The drawing under review shows one solid part. Ordinate dimensions are in mm from its lowest x, y, z. Coordinates: 2 decimals unless noted, no trailing zeros. Write each loop counter-clockwise with the first axis right and the second up, starting at its lowest first coordinate (ties: lowest second). Pieces come first, ordered by that corner, then holes.
Q1. Take a section at A-A (z = 10). Give the boundary of the cut face in (x, y), and give its area (3 significant figures).
Q2. Insertion check: pin 1 (3.5 mm diameter, centred on x = 10, z = 17, fed in from +Y); pin 2 (2.5 mm diameter, centred on x = 3, z = 10, fed in from +Y) (3 decimals). Each pin has a flat end and moves straight along its axis. Give the tip position at first contact, or say it passes through.
Q3. Mouldability with a two-part tool opening along Z and no side actions: class the marked faces 1, 2 and 3 as pulls with the +Z half, pulls with the -Z half, needs draft (parallel to the pull), parting line crosses it, or undercut.
Q4. Take a section at C-C (x = 10). Give the boundary of the cut face in (y, z).
Q5. Take a section at B-B (x = 17). Give the boundary of the cut face in (y, z), and give its area (3 significant figures).
Q6. Take a section at D-D (y = 1.5). Give the boundary of the cut face in (x, z).
Q7. For probe 1 along X at (y, z) = (1.5, 10); probe 2 along X at (y, z) = (1.45, 17.25), list the stretches that pass through material, from the lowest coordinate up.
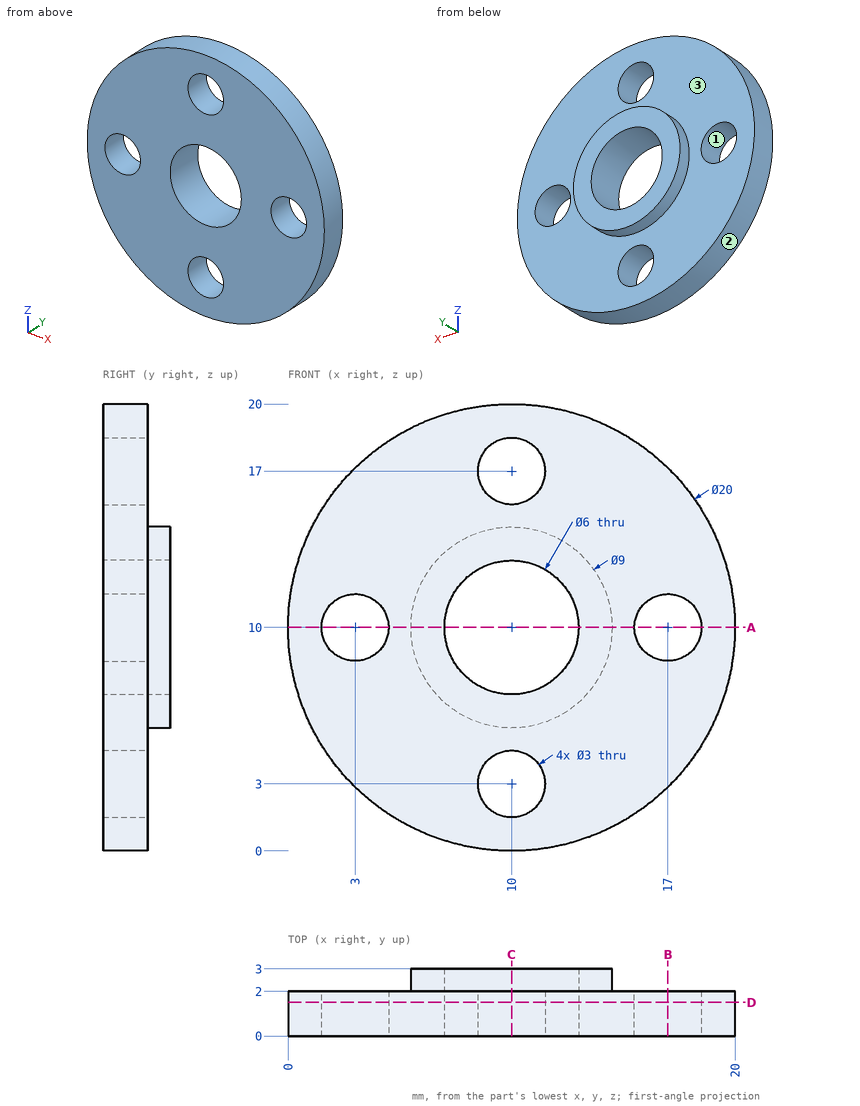
Response:
1. outline: (0, 0) - (1.5, 0) - (1.5, 2) - (0, 2) - close; (4.5, 0) - (7, 0) - (7, 3) - (5.5, 3) - (5.5, 2) - (4.5, 2) - close; (13, 0) - (15.5, 0) - (15.5, 2) - (14.5, 2) - (14.5, 3) - (13, 3) - close; (18.5, 0) - (20, 0) - (20, 2) - (18.5, 2) - close
1. area: 19.0 mm2
2. pin 1: stops at y = 2
2. pin 2: passes through
3. face 1: undercut
3. face 2: parting line crosses it
3. face 3: needs draft
4. outline: (0, 0) - (2, 0) - (2, 1.5) - (0, 1.5) - close; (0, 4.5) - (2, 4.5) - (2, 5.5) - (3, 5.5) - (3, 7) - (0, 7) - close; (0, 13) - (3, 13) - (3, 14.5) - (2, 14.5) - (2, 15.5) - (0, 15.5) - close; (0, 18.5) - (2, 18.5) - (2, 20) - (0, 20) - close
5. outline: (0, 2.86) - (2, 2.86) - (2, 8.5) - (0, 8.5) - close; (0, 11.5) - (2, 11.5) - (2, 17.14) - (0, 17.14) - close
5. area: 22.6 mm2
6. outline: circle Ø20 at (10, 10); hole circle Ø3 at (3, 10); hole circle Ø6 at (10, 10); hole circle Ø3 at (10, 3); hole circle Ø3 at (10, 17); hole circle Ø3 at (17, 10)
7. probe 1: x = 0 to 1.5, 4.5 to 7, 13 to 15.5, 18.5 to 20
7. probe 2: x = 3.11 to 8.52, 11.48 to 16.89
